from build123d import *

# Parameters (mm, degrees)
SKETCH2_R                            = 4.25
BOSS_EXTRUDE1_DEPTH                  = 30
SKETCH3_R                            = 11.25
SKETCH3_R_2                          = 5.25
SKETCH3_R_3                          = 4.25
CUT_EXTRUDE1_DEPTH                   = 5
CUT_EXTRUDE2_START                   = -5
SKETCH3_3_R                          = 5.25
SKETCH3_3_R_2                        = 4.25
CUT_EXTRUDE2_DEPTH                   = 10.6
SKETCH4_R                            = 2.4
CUT_EXTRUDE3_DEPTH                   = 56.118055118
SKETCH5_R                            = 1.3
CUT_EXTRUDE4_DEPTH                   = 6
SKETCH5_3_R                          = 1.3
BOSS_EXTRUDE2_DEPTH                  = 3.6
BOSS_EXTRUDE3_DEPTH                  = 15
BOSS_EXTRUDE3_DIRECTION_2_REACH      = 61.102
BOSS_EXTRUDE3_DIRECTION_2_END_RADIUS = 13
CUT_EXTRUDE5_START                   = -1.2
CUT_EXTRUDE5_DEPTH                   = 3.3


with BuildPart() as part:
    # Sketch2 → Boss-Extrude1 (new body)
    with BuildSketch(Plane(origin=(0, 0, 0), x_dir=(1, 0, 0), z_dir=(0, 1, 0))):
        with BuildLine():
            Line((0, 17), (0, -17))
            Line((0, -17), (5, -17))
            Line((5, -17), (5, -7))
            Line((5, -7), (24.04554885, -7))
            ThreePointArc((24.04554885, -7), (48, 0), (24.04554885, 7))
            Line((24.04554885, 7), (5, 7))
            Line((5, 7), (5, 17))
            Line((5, 17), (0, 17))
        make_face()
        with Locations(Location((35, 0, 0), (0, 0, 270))):
            Circle(SKETCH2_R, mode=Mode.SUBTRACT)
    extrude(amount=BOSS_EXTRUDE1_DEPTH)

    # Sketch3 → Cut-Extrude1 (cut)
    with BuildSketch(Plane.XZ):
        with Locations(Location((35, 0, 0), (0, 0, 270))):
            Circle(SKETCH3_R)
        with Locations((35, 0)):
            Circle(SKETCH3_R_2, mode=Mode.SUBTRACT)
        with Locations((35, 0)):
            Circle(SKETCH3_R_2)
        with Locations(Location((35, 0, 0), (0, 0, 270))):
            Circle(SKETCH3_R_3, mode=Mode.SUBTRACT)
    extrude(amount=-CUT_EXTRUDE1_DEPTH, mode=Mode.SUBTRACT)

    # Sketch3<3> → Cut-Extrude2 (cut)
    with BuildSketch(Plane.XZ.offset(CUT_EXTRUDE2_START)):
        with Locations(Location((35, 0, 0), (0, 0, 270))):
            Circle(SKETCH3_3_R)
        with Locations(Location((35, 0, 0), (0, 0, 270))):
            Circle(SKETCH3_3_R_2, mode=Mode.SUBTRACT)
    extrude(amount=-CUT_EXTRUDE2_DEPTH, mode=Mode.SUBTRACT)

    # Sketch4 → Cut-Extrude3 (cut, through all)
    with BuildSketch(Plane(origin=(5, 0, 0), x_dir=(0, 0, -1), z_dir=(1, 0, 0))):
        with Locations((12.17186788, 24.363439063)):
            Circle(SKETCH4_R)
        with Locations((12.17186788, 6.363439063)):
            Circle(SKETCH4_R)
        with Locations((-11.82813212, 6.363439063)):
            Circle(SKETCH4_R)
        with Locations((-11.82813212, 24.363439063)):
            Circle(SKETCH4_R)
    extrude(amount=-CUT_EXTRUDE3_DEPTH, mode=Mode.SUBTRACT)

    # Sketch5 → Cut-Extrude4 (cut)
    with BuildSketch(Plane.XZ.offset(-5)):
        with Locations(Location((35, 8, 0), (0, 0, 270))):
            Circle(SKETCH5_R)
        with Locations(Location((35, -8, 0), (0, 0, 270))):
            Circle(SKETCH5_R)
    extrude(amount=-CUT_EXTRUDE4_DEPTH, mode=Mode.SUBTRACT)

    # Sketch5<3> → Boss-Extrude2 (add)
    with BuildSketch(Plane.XZ.offset(-5)):
        with Locations(Location((27, 0, 0), (0, 0, 270))):
            Circle(SKETCH5_3_R)
        with Locations(Location((43, 0, 0), (0, 0, 270))):
            Circle(SKETCH5_3_R)
    extrude(amount=BOSS_EXTRUDE2_DEPTH)


with BuildPart() as boss_extrude3_tool:
    # Sketch7 → Boss-Extrude3 (new body)
    with BuildSketch(Plane(origin=(48, 0, 0), x_dir=(0, 0, -1), z_dir=(1, 0, 0))):
        Polygon((-5, 30), (5, 30), (7, 26.535898385), (-7, 26.535898385), align=None)
    extrude(amount=BOSS_EXTRUDE3_DEPTH)


with BuildPart() as part_1:
    add(part.part)


with BuildPart() as part_2:
    # Boss-Extrude3: joined with boss_extrude3_tool
    add(part_1.part.fuse(boss_extrude3_tool.part, tol=0.00001))

    # Boss-Extrude3 direction 2: up to this cylinder (the profile starts outside it)
    boss_extrude3_direction_2_end = Plane(origin=(35, 28.171724, 0), z_dir=(0, -1, 0)) * Cylinder(BOSS_EXTRUDE3_DIRECTION_2_END_RADIUS, 149.204, mode=Mode.PRIVATE)
    # Sketch7 → Boss-Extrude3 direction 2 (add, up to the surface)
    with BuildSketch(Plane(origin=(48, 0, 0), x_dir=(0, 0, -1), z_dir=(1, 0, 0)), mode=Mode.PRIVATE) as boss_extrude3_direction_2_sk1:
        Polygon((-5, 30), (5, 30), (7, 26.535898385), (-7, 26.535898385), align=None)
    boss_extrude3_direction_2_tool1 = extrude(boss_extrude3_direction_2_sk1.sketch, amount=-BOSS_EXTRUDE3_DIRECTION_2_REACH, mode=Mode.PRIVATE) - boss_extrude3_direction_2_end
    add(boss_extrude3_direction_2_tool1.solids().sort_by_distance((48, 28.171724, 0))[0])
    add(boss_extrude3_direction_2_tool1.solids().sort_by_distance((48, 28.171724, 0))[1])

    # Sketch9 → Cut-Extrude5 (cut)
    with BuildSketch(Plane(origin=(48, 0, 0), x_dir=(0, 0, -1), z_dir=(1, 0, 0)).offset(CUT_EXTRUDE5_START)):
        with BuildLine():
            Line((3.15, 30.472989279), (3.15, 9.535898385))
            ThreePointArc((3.15, 9.535898385), (0, 6.385898385), (-3.15, 9.535898385))
            Line((-3.15, 9.535898385), (-3.15, 30.472989279))
            ThreePointArc((-3.15, 30.472989279), (0, 33.622989279), (3.15, 30.472989279))
        make_face()
    extrude(amount=-CUT_EXTRUDE5_DEPTH, mode=Mode.SUBTRACT)


solid = part_2.part
Can you work these out from the model? Positions are in its coordinate system, mm. A direction names the side the tool comes from. Give positions to 0.01 mm unless a question says otherwise; leave off trailing zeros. Write each loop counter-clockwise with the first axis right and the second up, starting at its lowest first coordinate (ties: lowest second). Pieces come first, ordered by that corner, then holes. Notation, with made-up numbers: M -27,8 L 13,8 A7 ccw 13,20 Z; hole C 34,83 d6. An arc over 180 degrees is marked long. Answer in a Markdown table with one row per item. Add a question column.
Item 1: On a 3-axis mill with a long thin cutter (end or side, diameter ignored), from which of +Z, -Z, +X, -X, +Y, -Y can I reach the whole of each face in a straight line? I mean faces 1 (the cylindrical face through (45.173, 6.387, -0.069)), 2 (the cylindrical face through (44.29, 3.23, 0.17)), 3 (the cylindrical face through (2.535, 4.234, -13.279)). Say none if no direction works.
Item 2: Imagine slicing it at A-A, the plane x = 35. Write out the boundary of the cut face in (y, z).
Item 3: Please list where these lines run through material, in increasing order: L1, parallel to Z at x = 35, y = 25.25; L2, parallel to X at y = 6, z = -8; L3, parallel to X at y = 1.1, z = 0.
Item 4: Imagine slicing it at B-B, the plane y = 14. Write out the boundary of the cut face in (x, z), plus the area to 3 significant figures.
Item 5: For pin 1 Ø1.3 at (x, z) = (35.5, -7.5) entering from -Y; pin 2 Ø3 at (y, z) = (22, -10) entering from +X; pin 3 Ø11 at (x, z) = (38.5, 3.5) entering from -Y, each with a flat end and sliding along its axis, tell me the tip position at first contact or that it passes through.
Item 6: Imagine slicing it at D-D, the plane z = 10.5. Write out the boundary of the cut face in (x, y), plus the area to 3 significant figures.
Item 7: We'd pull the mould along Z, two halves only. Please class faces 4 (the flat face through (54.597, 28.292, -5.986)), 5 (the flat face through (55, 26.536, 0)), 6 (the flat face through (45, 20, 3.15)), 7 (the cylindrical face through (44.486, 2.465, -6.048)): released by +Z, released by -Z, zero draft, split by the parting line, or undercut.
Evaluation:
| question | item | result |
|---|---|---|
| 1 | face 1 | +Y |
| 1 | face 2 | -Y |
| 1 | face 3 | -X |
| 2 | outline | M 0,-13 L 30,-13 L 30,-4.25 L 15.6,-4.25 L 15.6,-5.25 L 5,-5.25 L 5,-6.7 L 11,-6.7 L 11,-9.3 L 5,-9.3 L 5,-11.25 L 0,-11.25 Z; M 0,11.25 L 5,11.25 L 5,9.3 L 11,9.3 L 11,6.7 L 5,6.7 L 5,5.25 L 15.6,5.25 L 15.6,4.25 L 30,4.25 L 30,13 L 0,13 Z |
| 3 | L1 | z = -13 to -4.25, 4.25 to 13 |
| 3 | L2 | x = 0 to 5, 24.75 to 33.7, 36.3 to 45.25 |
| 3 | L3 | x = 0 to 23.75, 46.25 to 48 |
| 4 | outline | M 0,-17 L 5,-17 L 5,-7 L 24.05,-7 A13 ccw long 24.05,7 L 5,7 L 5,17 L 0,17 Z; hole C 35,0 d10.5; hole M 43.5,-3.15 L 46.8,-3.15 L 46.8,3.15 L 43.5,3.15 Z |
| 4 | area | 841 mm² |
| 5 | pin 1 | stops at y = 5 |
| 5 | pin 2 | stops at x = 44.84 |
| 5 | pin 3 | stops at y = 1.4 |
| 6 | outline | M 0,0 L 5,0 L 5,4.36 L 0,4.36 Z; M 0,8.36 L 5,8.36 L 5,22.36 L 0,22.36 Z; M 0,26.36 L 5,26.36 L 5,30 L 0,30 Z; M 27.34,0 L 30.96,0 L 30.96,5 L 39.04,5 L 39.04,0 L 42.66,0 L 42.66,30 L 27.34,30 Z |
| 6 | area | 530 mm² |
| 7 | face 4 | released by -Z |
| 7 | face 5 | zero draft |
| 7 | face 6 | undercut |
| 7 | face 7 | undercut |
